Model file for the job. Use its own axes, mm. Round coordinates to 2 decimals unless told otherwise and drop trailing zeros. Order: outer loops, then holes, each group sorted by start corner. A loop starts at its lowest first (then second) coordinate and runs counter-clockwise, first axis right, second up. Notation, with made-up numbers: (-12.5, 87) - (28.5, 87) arc R25 ccw to (28.5, 113) - close; hole circle Ø6 at (-17.5, 55.5). An arc over 180 degrees is marked (long way). Use one line per item in the form item = value.
from build123d import *

# Parameters (mm, degrees)
F0_R     = 50.8
F0_R_2   = 11.049
F1_DEPTH = 4.7625
F2_R     = 4.76249


# Not quite as in the source:
# - a fillet or chamfer is up to 0.001 mm smaller than in the source, because OpenCascade refuses the exact size


with BuildPart() as f1:
    # F0 (on Top) → F1 (new body, symmetric)
    with BuildSketch(Plane.XY):
        Circle(F0_R)
        with BuildLine():
            ThreePointArc((11.049, -31.75), (-7.8128228253, -39.5628228253), (0, -20.701))
            ThreePointArc((0, -20.701), (7.8128228253, -23.9371771747), (11.049, -31.75))
        make_face(mode=Mode.SUBTRACT)
        with Locations((-31.75, 0)):
            Circle(F0_R_2, mode=Mode.SUBTRACT)
        with BuildLine():
            ThreePointArc((0, 11.049), (7.8128228253, 7.8128228253), (11.049, 0))
            ThreePointArc((11.049, 0), (7.8128228253, -7.8128228253), (0, -11.049))
            ThreePointArc((0, -11.049), (-7.8128228253, -7.8128228253), (-11.049, 0))
            ThreePointArc((-11.049, 0), (-7.8128228253, 7.8128228253), (0, 11.049))
        make_face(mode=Mode.SUBTRACT)
        with BuildLine():
            ThreePointArc((42.799, 0), (31.75, -11.049), (20.701, 0))
            ThreePointArc((20.701, 0), (31.75, 11.049), (42.799, 0))
        make_face(mode=Mode.SUBTRACT)
        with BuildLine():
            ThreePointArc((11.049, 31.75), (7.8128228253, 23.9371771747), (0, 20.701))
            ThreePointArc((0, 20.701), (-7.8128228253, 39.5628228253), (11.049, 31.75))
        make_face(mode=Mode.SUBTRACT)
    extrude(amount=F1_DEPTH, both=True)

    # F2 (radius 4.7625 in the source; OpenCascade refuses exactly that, so slightly less here)
    f2_edges = [f1.edges().sort_by_distance(p)[0] for p in [
        (-50.8, 0, -4.7625),
        (50.8, 0, 0),
        (-50.8, 0, 4.7625),
    ]]
    fillet(f2_edges, radius=F2_R)


solid = f1.part
(1) Slice it at B-B on y = -5.5. Count the separate pieces of the cut face and the enclosed holes in it, then the cut area to 3 significant figures.
Report:
separate_pieces = 4
enclosed_holes = 0
area = 395 mm2
(2) Probe probe 1 along Y at (x, z) = (-2.5, -1.5); probe 2 along Y at (x, z) = (1, -3.25); probe 3 along X at (y, z) = (-1.5, -1.25). List the from-to ranges inside material, lowest first. Write a range as [from, to].
Report:
probe_1 = [-50.5, -42.51], [-20.99, -10.76], [10.76, 20.99], [42.51, 50.5]
probe_2 = [-49.51, -42.75], [-20.75, -11], [11, 20.75], [42.75, 49.51]
probe_3 = [-50.61, -42.7], [-20.8, -10.95], [10.95, 20.8], [42.7, 50.61]
(3) Pin check, flat tips, straight feed: pin 1 (3 mm diameter, centred on x = 36.5, y = -35, fed in from +Z); pin 2 (13.5 mm diameter, centred on x = -31.75, y = 0, fed in from +Z); pin 3 (2 mm diameter, centred on x = 38, z = -2.5, fed in from +Y); pin 4 (1.5 mm diameter, centred on x = 15.5, z = -2.5, fed in from -Y). Stop position of each tip, or through.
Report:
pin_1 = 3.67
pin_2 = through
pin_3 = 34.02
pin_4 = -48.11
(4) Pull direction X, two halves, no side cores. Call faces 1 (the face through (10, -10, 4.762)), 2 (the face through (-11.04, 31.26, -0.07)): released by +X, released by -X, zero draft, split by the parting line, or undercut.
Report:
face_1 = zero draft
face_2 = undercut
(5) Slice it at D-D on z = 3.25. Give the cut face in (x, y), then the cut area to 3 significant figures.
Report:
outline = circle Ø99.04 at (0, 0); hole circle Ø22.1 at (-31.75, 0); hole circle Ø22.1 at (0, -31.75); hole circle Ø22.1 at (0, 0); hole circle Ø22.1 at (0, 31.75); hole circle Ø22.1 at (31.75, 0)
area = 5,790 mm2
(6) Slice it at A-A on z = -2.5. Give the cut face in (x, y).
Report:
outline = circle Ø100.18 at (0, 0); hole circle Ø22.1 at (-31.75, 0); hole circle Ø22.1 at (0, -31.75); hole circle Ø22.1 at (0, 0); hole circle Ø22.1 at (0, 31.75); hole circle Ø22.1 at (31.75, 0)
